```python
from build123d import *

# Parameters (mm, degrees)
SKETCH10_W          = 50
SKETCH10_H          = 50
BOSS_EXTRUDE7_DEPTH = 5
SKETCH9_W           = 50
SKETCH9_H           = 50
BOSS_EXTRUDE8_DEPTH = 5
SKETCH11_R          = 0.75
CUT_EXTRUDE5_DEPTH  = 5
CHAMFER1_SIZE       = 2
SKETCH12_R          = 1
CUT_EXTRUDE6_DEPTH  = 10
SKETCH14_R          = 0.75
CUT_EXTRUDE8_DEPTH  = 5
BOSS_EXTRUDE9_DEPTH = 2
FILLET1_R           = 1
FILLET2_R           = 25


# Some blends are built 0.0001 mm under size
with BuildPart() as part:
    # Sketch10 → Boss-Extrude7 (new body)
    with BuildSketch(Plane(origin=(0, 0, 0), x_dir=(-1, 0, 0), z_dir=(0, 0, -1))):
        with Locations((-42.5, 20.5)):
            Rectangle(SKETCH10_W, SKETCH10_H)
    extrude(amount=-BOSS_EXTRUDE7_DEPTH)

    # Sketch9 → Boss-Extrude8 (add)
    with BuildSketch(Plane(origin=(0, 0, 0), x_dir=(-1, 0, 0), z_dir=(0, 0, -1))):
        with Locations((-42.5, 20.5)):
            Rectangle(SKETCH9_W, SKETCH9_H)
        with BuildLine():
            Line((-59.2, 24.3), (-48.011787453, 24.5))
            ThreePointArc((-48.011787453, 24.5), (-46.919880362, 24.919880362), (-46.5, 26.011787453))
            Line((-46.5, 26.011787453), (-46.3, 37.2))
            ThreePointArc((-46.3, 37.2), (-42.5, 41), (-38.7, 37.2))
            Line((-38.7, 37.2), (-38.5, 26.011787453))
            ThreePointArc((-38.5, 26.011787453), (-38.080119638, 24.919880362), (-36.988212547, 24.5))
            Line((-36.988212547, 24.5), (-25.8, 24.3))
            ThreePointArc((-25.8, 24.3), (-22, 20.5), (-25.8, 16.7))
            Line((-25.8, 16.7), (-36.988212547, 16.5))
            ThreePointArc((-36.988212547, 16.5), (-38.080119638, 16.080119638), (-38.5, 14.988212547))
            Line((-38.5, 14.988212547), (-38.7, 3.8))
            ThreePointArc((-38.7, 3.8), (-42.5, 0), (-46.3, 3.8))
            Line((-46.3, 3.8), (-46.5, 14.988212547))
            ThreePointArc((-46.5, 14.988212547), (-46.919880362, 16.080119638), (-48.011787453, 16.5))
            Line((-48.011787453, 16.5), (-59.2, 16.7))
            ThreePointArc((-59.2, 16.7), (-63, 20.5), (-59.2, 24.3))
        make_face(mode=Mode.SUBTRACT)
    extrude(amount=BOSS_EXTRUDE8_DEPTH)

    # Sketch11 → Cut-Extrude5 (cut)
    with BuildSketch(Plane(origin=(0, 0, 0), x_dir=(-1, 0, 0), z_dir=(0, 0, -1))):
        with Locations((-59, 20.5)):
            Circle(SKETCH11_R)
        with Locations(Location((-26, 20.5, 0), (0, 0, 180))):
            Circle(SKETCH11_R)
    extrude(amount=-CUT_EXTRUDE5_DEPTH, mode=Mode.SUBTRACT)

    # Chamfer1
    chamfer1_edges = [part.edges().sort_by_distance(p)[0] for p in [
        (42.5, 45.5, 5),
        (67.5, 20.5, -5),
        (42.5, -4.5, -5),
        (17.5, 20.5, -5),
        (42.5, 45.5, -5),
        (42.5, -4.5, 5),
    ]]
    chamfer(chamfer1_edges, length=CHAMFER1_SIZE)

    # Sketch12 → Cut-Extrude6 (cut)
    with BuildSketch(Plane.XY.offset(5)):
        with Locations((42.5, 20.5)):
            Circle(SKETCH12_R)
    extrude(amount=-CUT_EXTRUDE6_DEPTH, mode=Mode.SUBTRACT)

    # Sketch14 → Cut-Extrude8 (cut)
    with BuildSketch(Plane.XY.offset(5)):
        with Locations((42.5, 36.5)):
            Circle(SKETCH14_R)
        with Locations((42.5, 4.5)):
            Circle(SKETCH14_R)
    extrude(amount=-CUT_EXTRUDE8_DEPTH, mode=Mode.SUBTRACT)

    # Sketch15 → Boss-Extrude9 (add)
    with BuildSketch(Plane.XY.offset(5)):
        with BuildLine():
            Line((40, 0.112312602), (45, 0.112312602))
            ThreePointArc((45, 0.112312602), (46, -0.887687398), (45, -1.887687398))
            Line((45, -1.887687398), (40, -1.887687398))
            ThreePointArc((40, -1.887687398), (39, -0.887687398), (40, 0.112312602))
        make_face()
    extrude(amount=BOSS_EXTRUDE9_DEPTH)

    # Fillet1
    fillet1_edges = [part.edges().sort_by_distance(p)[0] for p in [
        (39, -0.887687398, 7),
        (42.5, -1.887687398, 7),
        (46, -0.887687398, 7),
        (42.5, 0.112312602, 7),
    ]]
    fillet(fillet1_edges, radius=FILLET1_R - 0.0001)  # a hair under: the kernel refuses the full size

    # Fillet2
    # the kernel refuses this fillet: 25 mm, written as the material it takes off along each edge
    with BuildSketch(Plane(origin=(17.5, 45.5, -65.5), x_dir=(0, -1, 0), z_dir=(0, 0, 1)), Plane(origin=(67.5, 45.5, 65.5), x_dir=(0, -1, 0), z_dir=(0, 0, -1))) as fillet2_piece_1:
        with BuildLine():
            CenterArc((FILLET2_R, FILLET2_R), FILLET2_R, 180, 90)
            Line((0, FILLET2_R), (0, 0))
            Line((0, 0), (FILLET2_R, 0))
        make_face()
    extrude(amount=131, mode=Mode.SUBTRACT)
    with BuildSketch(Plane(origin=(67.5, -4.5, 65.5), x_dir=(0, 1, 0), z_dir=(0, 0, -1)), Plane(origin=(17.5, -4.5, -65.5), x_dir=(0, 1, 0), z_dir=(0, 0, 1))) as fillet2_piece_2:
        with BuildLine():
            CenterArc((FILLET2_R, -FILLET2_R), FILLET2_R, 90, 90)
            Line((0, -FILLET2_R), (0, 0))
            Line((0, 0), (FILLET2_R, 0))
        make_face()
    extrude(amount=131, mode=Mode.SUBTRACT)


solid = part.part
```
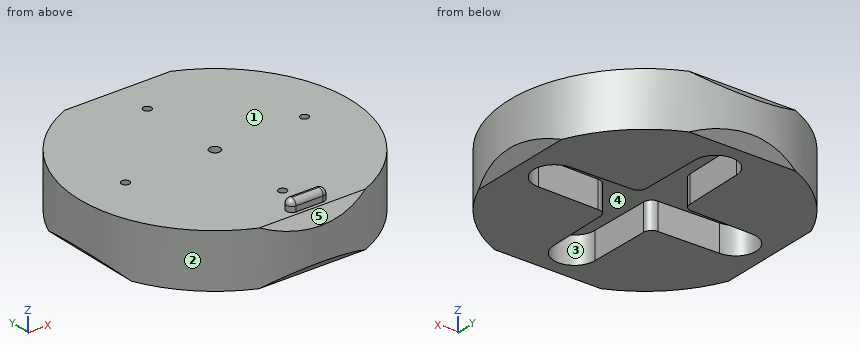
The listing builds one solid part. Answer for the finished solid, in the listing's coordinates (mm). Face numbers are marked on the shaded views. A direction names the side the tool comes from. Give positions to 0.01 mm unless a question says otherwise; leave off trailing zeros. Order: outer loops, then holes, each group sorted by start corner. A loop starts at its lowest first (then second) coordinate and runs counter-clockwise, first axis right, second up.
Item 1: The part is cut by section B-B, the plane y = 36.5. Give the vertices of the cut face in (x, z).
From the geometry:
outline: (23.29, -5) - (38.69, -5) - (38.69, 0) - (41.75, 0) - (41.75, 5) - (23.29, 5) - close; (43.25, 0) - (46.31, 0) - (46.31, -5) - (61.71, -5) - (61.71, 5) - (43.25, 5) - close
Item 2: The part is cut by section C-C, the plane x = 54. Give the vertices of the cut face in (y, z), and give its area (3 significant figures).
From the geometry:
outline: (-1.7, -5) - (16.61, -5) - (16.61, 0) - (24.39, 0) - (24.39, -5) - (42.7, -5) - (42.7, 5) - (-1.7, 5) - close
area: 405 mm2
Item 3: The part is cut by section A-A, the plane y = 20.5. Give the vertices of the cut face in (x, z), and give its area (3 significant figures).
From the geometry:
outline: (17.5, -3) - (19.5, -5) - (22, -5) - (22, 0) - (25.25, 0) - (25.25, 5) - (17.5, 5) - close; (26.75, 0) - (41.5, 0) - (41.5, 5) - (26.75, 5) - close; (43.5, 0) - (58.25, 0) - (58.25, 5) - (43.5, 5) - close; (59.75, 0) - (63, 0) - (63, -5) - (65.5, -5) - (67.5, -3) - (67.5, 5) - (59.75, 5) - close
area: 266 mm2
Item 4: Find the intervals of material crossed by probe 1 along Y at (x, z) = (42.5, 2.15); probe 2 along Z at (x, y) = (54.5, -1); probe 3 along X at (y, z) = (36.5, 3.8), in increasing order.
From the geometry:
probe 1: y = -4.5 to 3.75, 5.25 to 19.5, 21.5 to 35.75, 37.25 to 45.5
probe 2: z = -5 to 5
probe 3: x = 23.29 to 41.75, 43.25 to 61.71
Item 5: The part is cut by section D-D, the plane y = 8.5. Give the vertices of the cut face in (x, z), and give its area (3 significant figures).
From the geometry:
outline: (20.57, -5) - (38.62, -5) - (38.62, 0) - (46.38, 0) - (46.38, -5) - (64.43, -5) - (64.43, 5) - (20.57, 5) - close
area: 400 mm2
Item 6: Which of the six approach directions +Z, -Z, +X, -X, +Y, -Y give full straight-line access (tool end or side, diameter ignored) to the marked faces 4 and 5?
From the geometry:
face 4: -Z
face 5: +Z, +X, -X, -Y
Item 7: Given pin 1 Ø1.5 at (x, y) = (57, 17) entering from +Z; pin 2 Ø6 at (y, z) = (38, 4.5) entering from +X; pin 3 Ø3 at (x, z) = (43, -3) entering from -Y; pin 4 Ø3 at (x, z) = (54.5, 2.5) entering from +Y, each flat-ended and moving along its own axis, determine where each tip first touches the part or whether it passes through.
From the geometry:
pin 1: stops at z = 5
pin 2: stops at x = 62.87
pin 3: stops at y = -4.5
pin 4: stops at y = 43.19
Item 8: For a pull along X with two mould halves and no side action, classify the marked faces 1, 2 and 3 as pulls with the +X half, pulls with the -X half, needs draft (parallel to the pull), parting line crosses it, or undercut.
From the geometry:
face 1: needs draft
face 2: parting line crosses it
face 3: undercut
